Autodesk Inventor part; units mm, degrees
ref_plane "YZ Plane" through (0, 0, 0) normal (1, 0, 0) x (0, 1, 0)
ref_plane "XZ Plane" through (0, 0, 0) normal (0, 1, 0) x (-1, 0, 0)
ref_plane "XY Plane" through (0, 0, 0) normal (0, 0, 1) x (1, 0, 0)
sketch "Sketch1" plane through (0, 0, 0) normal (0, 0, 1) x (1, 0, 0)
  line L0 (0, 0) -> (220, 0)
  line L1 (220, 0) -> (220, 220)
  line L2 (220, 220) -> (0, 220)
  line L3 (0, 220) -> (0, 0)
  line L4 (5.5, 214.5) -> (214.5, 214.5) construction
  line L5 (214.5, 214.5) -> (214.5, 5.5) construction
  line L6 (214.5, 5.5) -> (5.5, 5.5) construction
  line L7 (5.5, 5.5) -> (5.5, 214.5) construction
  circle A0 centre (5.5, 5.5) radius 1.6
  circle A1 centre (5.5, 214.5) radius 1.6
  circle A2 centre (214.5, 214.5) radius 1.6
  circle A3 centre (214.5, 5.5) radius 1.6
  line L8 (165, 87.2183) -> (132.7817, 55)
  line L9 (132.7817, 55) -> (87.2183, 55)
  line L10 (87.2183, 55) -> (55, 87.2183)
  line L11 (55, 87.2183) -> (55, 132.7817)
  line L12 (55, 132.7817) -> (87.2183, 165)
  line L13 (132.7817, 165) -> (165, 132.7817)
  line L14 (165, 132.7817) -> (165, 87.2183)
  line L15 (150, 126.5685) -> (150, 93.4315)
  line L16 (150, 93.4315) -> (126.5685, 70)
  line L17 (126.5685, 70) -> (93.4315, 70)
  line L18 (93.4315, 70) -> (70, 93.4315)
  line L19 (70, 93.4315) -> (70, 126.5685)
  line L20 (70, 126.5685) -> (93.4315, 150)
  line L21 (93.4315, 150) -> (126.5685, 150)
  line L22 (126.5685, 150) -> (150, 126.5685)
  line L23 (205, 205) -> (205, 15)
  line L24 (205, 15) -> (15, 15)
  line L25 (15, 15) -> (15, 205)
  line L26 (102.5, 165) -> (102.5, 205)
  line L27 (117.5, 205) -> (117.5, 165)
  line L28 (15, 205) -> (102.5, 205)
  line L29 (117.5, 205) -> (205, 205)
  line L30 (87.2183, 165) -> (102.5, 165)
  line L31 (117.5, 165) -> (132.7817, 165)
  point P0 (214.5, 110)
  point P1 (220, 110)
  point P2 (110, 214.5)
  point P3 (110, 220)
  point P4 (110, 110)
  point P5 (110, 110)
  dimension "d0" = 220
  dimension "d1" = 220
  dimension "d2" = 209
  dimension "d3" = 209
  dimension "d4" = 3.2
  dimension "d5" = 3.2
  dimension "d6" = 3.2
  dimension "d7" = 3.2
  dimension "d9" = 15
  dimension "d10" = 15
  dimension "d11" = 15
  dimension "d12" = 15
  dimension "d13" = 15
  dimension "d14" = 80
  dimension "d15" = 7.5
extrude "Extrusion1" add sketch "Sketch1" along normal blind 6.5
sketch "Sketch2" plane through (0, 0, 6.5) normal (0, 0, 1) x (1, 0, 0)
  line L0 (205, 205) -> (205, 15)
  line L1 (205, 15) -> (15, 15)
  line L2 (15, 15) -> (15, 205)
  line L3 (55, 87.2183) -> (87.2183, 55)
  line L4 (132.7817, 55) -> (165, 87.2183)
  line L5 (0, 220) -> (0, 0)
  line L6 (65.8058, 76.4124) -> (15, 25.6066)
  line L7 (76.4124, 65.8058) -> (25.6066, 15)
  line L8 (143.5876, 65.8058) -> (194.3934, 15)
  line L9 (154.1942, 76.4124) -> (205, 25.6066)
  line L10 (205, 25.6066) -> (205, 15)
  line L11 (205, 15) -> (194.3934, 15)
  line L12 (15, 25.6066) -> (15, 15)
  line L13 (15, 15) -> (25.6066, 15)
  line L14 (15, 15) -> (71.1091, 71.1091) construction
  line L15 (148.8909, 71.1091) -> (205, 15) construction
  line L16 (65.8058, 76.4124) -> (76.4124, 65.8058)
  line L17 (143.5876, 65.8058) -> (154.1942, 76.4124)
  dimension "d18" = 15
  dimension "d19" = 15
  dimension "d20" = 7.5
  dimension "d21" = 7.5
extrude "Extrusion2" add sketch "Sketch2" against normal blind 6.5
sketch "Sketch4" plane through (0, 0, 6.5) normal (0, 0, 1) x (1, 0, 0)
  line L0 (93.4315, 150) -> (126.5685, 150)
  line L1 (0, 0) -> (220, 0)
  line L2 (220, 0) -> (220, 220)
  line L3 (220, 220) -> (0, 220)
  line L4 (0, 220) -> (0, 0)
  line L5 (-23.9453, -6) -> (243.9453, -6) construction
  line L6 (-23.9453, -6) -> (110, 226) construction
  line L7 (110, 226) -> (243.9453, -6) construction
  circle A0 centre (110, 226) radius 2.75
  circle A1 centre (243.9453, -6) radius 2.75
  circle A2 centre (-23.9453, -6) radius 2.75
  arc A3 (-30.4405, -2.25) -> (-22.5946, -13.3774) centre (-23.9453, -6) ccw
  arc A4 (116.4952, 229.75) -> (103.5048, 229.75) centre (110, 226) ccw
  arc A5 (242.5946, -13.3774) -> (250.4405, -2.25) centre (243.9453, -6) ccw
  line L8 (122.1244, 220) -> (116.4952, 229.75)
  line L9 (103.5048, 229.75) -> (97.8756, 220)
  line L10 (0, 50.4744) -> (-30.4405, -2.25)
  line L11 (250.4405, -2.25) -> (220, 50.4744)
  line L12 (242.5946, -13.3774) -> (169.5256, 0)
  line L13 (-22.5946, -13.3774) -> (50.4744, 0)
  line L14 (0, 50.4744) -> (0, 0)
  line L15 (0, 0) -> (50.4744, 0)
  line L16 (169.5256, 0) -> (220, 0)
  line L17 (220, 50.4744) -> (220, 0)
  point P0 (110, 150)
  dimension "d30" = 5.5
  dimension "d31" = 5.5
  dimension "d32" = 5.5
  dimension "d33" = 15
  dimension "d34" = 15
  dimension "d35" = 15
  dimension "d36" = 6
  dimension "d37" = 6
extrude "Extrusion3" add sketch "Sketch4" against normal blind 6.5 contours L1 L13 A3 L10 L4 | L1 L2 L11 A5 L12 | L9 A4 L8 L3
chamfer "Chamfer1" distance 4 angle 45 16 edges at (25.6066, 15, 3.25) (15, 25.6066, 3.25) (76.4124, 65.8058, 3.25) (65.8058, 76.4124, 3.25) (194.3934, 15, 3.25) (205, 25.6066, 3.25) (143.5876, 65.8058, 3.25) (154.1942, 76.4124, 3.25) (117.5, 205, 3.25) (102.5, 205, 3.25) (117.5, 165, 3.25) (102.5, 165, 3.25) (205, 205, 3.25) (15, 205, 3.25) (0, 220, 3.25) (220, 220, 3.25)
sketch "Sketch5" plane through (0, 0, 6.5) normal (0, 0, 1) x (1, 0, 0)
  line L0 (117.5, 169) -> (117.5, 201)
  line L1 (28.435, 17.8284) -> (29.6066, 15)
  line L2 (15, 29.6066) -> (17.8284, 28.435)
  line L3 (102.5, 201) -> (102.5, 169)
  line L4 (93.4315, 150) -> (126.5685, 150)
  line L5 (0, 216) -> (4, 220)
  line L6 (220, 50.4744) -> (220, 216)
  line L7 (70, 126.5685) -> (150, 93.4315) construction
  line L8 (150, 126.5685) -> (70, 93.4315) construction
  line L9 (102.5, 150) -> (102.5, 106)
  line L10 (102.5, 106) -> (106, 102.5)
  line L11 (106, 102.5) -> (114, 102.5)
  line L12 (114, 102.5) -> (117.5, 106)
  line L13 (117.5, 106) -> (117.5, 150)
  circle A0 centre (110, 110) radius 1.5
  point P0 (0, 0)
  dimension "d43" = 3
  dimension "d44" = 8
  dimension "d45" = 7.5
  dimension "d46" = 7.5
extrude "Extrusion4" add sketch "Sketch5" against normal blind 6.5
chamfer "Chamfer2" distance 4 angle 45 2 edges at (102.5, 150, 3.25) (117.5, 150, 3.25)
sketch "Sketch6" plane through (0, 0, 6.5) normal (0, 0, 1) x (1, 0, 0)
  line L0 (50.4744, 0) -> (169.5256, 0)
  line L1 (107.5, 0) -> (107.5, 1.4434)
  line L2 (107.5, 1.4434) -> (110, 2.8868)
  line L3 (110, 2.8868) -> (112.5, 1.4434)
  line L4 (112.5, 1.4434) -> (112.5, 0)
  line L5 (107.5, 0) -> (112.5, 0)
  point P0 (0, 0)
  point P1 (110, 0)
  dimension "d52" = 5
extrude "Extrusion5" cut sketch "Sketch6" against normal through all
equation "\"d5\" = d4"
equation "\"d6\" = d4"
equation "\"d7\" = d4"
equation "\"d31\" = d30"
equation "\"d32\" = d30"
equation "\"d34\" = d33"
equation "\"d35\" = d33"
equation "\"d46\" = d45"
properties part number "heatbed_mount_v3" material "Plywood, Finish"
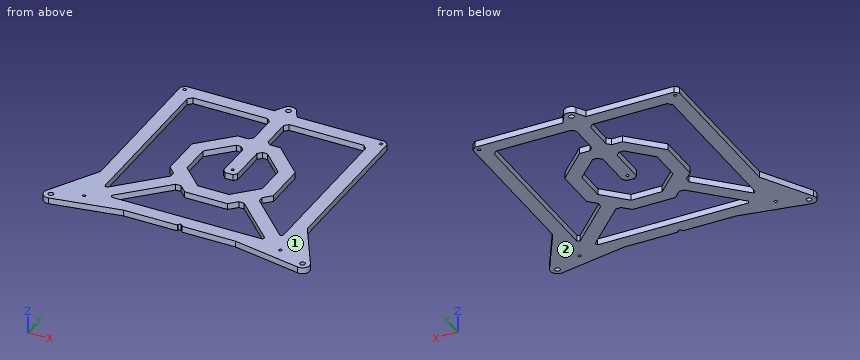
Check sheet for the modelled part. Datum: model origin and axes. Units: mm. Face numbers are marked on the shaded views. Round coordinates to 2 decimals unless told otherwise and drop trailing zeros. Order: outer loops, then holes, each group sorted by start corner. A loop starts at its lowest first (then second) coordinate and runs counter-clockwise, first axis right, second up. Notation, with made-up numbers: (-2.75, 78.25) - (27.25, 78.25) arc R12 cw to (27.25, 82.25) - close; hole circle Ø3 at (4.25, 82.5). An arc over 180 degrees is marked (long way). Write item = value, one per line.
Q1. Section check B-B (z = 1.75). State how many separate pieces and enclosed holes the cut face has, and give its area (3 significant figures).
Computed:
separate_pieces = 1
enclosed_holes = 12
area = 23,400 mm^2
Q2. Section check A-A (y = 191.5). Record the boundary of the cut face in (x, z).
Computed:
outline = (0, 0) - (15, 0) - (15, 6.5) - (0, 6.5) - close; (102.5, 0) - (117.5, 0) - (117.5, 6.5) - (102.5, 6.5) - close; (205, 0) - (220, 0) - (220, 6.5) - (205, 6.5) - close
Q3. Draft check along Z on the marked faces 1 and 2. Enter one of: pulls with the +Z half, pulls with the -Z half, needs draft (parallel to the pull), parting line crosses it, or undercut.
Computed:
face_1 = pulls with the +Z half
face_2 = pulls with the -Z half
Q4. Go/stop test with flat-tipped pins: pin 1 (3.5 mm diameter, centred on x = -23.95, y = -6, fed in from -Z); pin 2 (2 mm diameter, centred on x = 204.5, z = 3, fed in from +Y); pin 3 (3 mm diameter, centred on x = 119.5, z = 3, fed in from +Y); pin 4 (4 mm diameter, centred on x = 5.5, y = 214.5, fed in from -Z). Record where each tip stops, or that it passes through.
Computed:
pin_1 = through
pin_2 = 220
pin_3 = 227.14
pin_4 = 0
Q5. Thickness scan on line 1 along Y through (x, z) = (123, 5.5); line 2 along X through (y, z) = (115.5, 3.75); line 3 along X through (y, z) = (189, 3). Record the ranges inside material, lowest first.
Computed:
line_1 = 0 to 15, 55 to 70, 150 to 165, 205 to 220
line_2 = 0 to 15, 55 to 70, 102.5 to 117.5, 150 to 165, 205 to 220
line_3 = 0 to 15, 102.5 to 117.5, 205 to 220
